```python
from build123d import *

# Parameters (mm, degrees)
SALIENTE_EXTRUIR1_DEPTH = 0.8
CROQUIS5_R              = 5.15
CORTAR_EXTRUIR1_DEPTH   = 0.8
CROQUIS4_R              = 2.1
CORTAR_EXTRUIR2_DEPTH   = 0.8


with BuildPart() as part:
    # Croquis1 → Saliente-Extruir1 (new body)
    with BuildSketch(Plane.XY):
        with BuildLine():
            Line((-55.5, 86), (-55.5, 78))
            ThreePointArc((-55.5, 78), (-55.792893219, 77.292893219), (-56.5, 77))
            Line((-56.5, 77), (-58.5, 77))
            ThreePointArc((-58.5, 77), (-59.207106781, 76.707106781), (-59.5, 76))
            Line((-59.5, 76), (-59.5, -36))
            ThreePointArc((-59.5, -36), (-58.621320344, -38.121320344), (-56.5, -39))
            Line((-56.5, -39), (50.5, -39))
            ThreePointArc((50.5, -39), (52.621320344, -38.121320344), (53.5, -36))
            Line((53.5, -36), (53.5, 124))
            ThreePointArc((53.5, 124), (52.621320344, 126.121320344), (50.5, 127))
            Line((50.5, 127), (-56.5, 127))
            ThreePointArc((-56.5, 127), (-58.621320344, 126.121320344), (-59.5, 124))
            Line((-59.5, 124), (-59.5, 88))
            ThreePointArc((-59.5, 88), (-59.207106781, 87.292893219), (-58.5, 87))
            Line((-58.5, 87), (-56.5, 87))
            ThreePointArc((-56.5, 87), (-55.792893219, 86.707106781), (-55.5, 86))
        make_face()
    extrude(amount=SALIENTE_EXTRUIR1_DEPTH)

    # Croquis5 → Cortar-Extruir1 (cut)
    with BuildSketch(Plane.XY.offset(0.8)):
        Circle(CROQUIS5_R)
        with BuildLine():
            Line((-17.937391115, -1.5), (-12.787322824, -1.5))
            ThreePointArc((-12.787322824, -1.5), (-9.103999808, -9.103999808), (-1.5, -12.787322824))
            Line((-1.5, -12.787322824), (-1.5, -17.937391115))
            ThreePointArc((-1.5, -17.937391115), (-12.727922061, -12.727922061), (-17.937391115, -1.5))
        make_face()
        with BuildLine():
            Line((-17.937391115, 1.5), (-12.787322824, 1.5))
            ThreePointArc((-12.787322824, 1.5), (-9.103999808, 9.103999808), (-1.5, 12.787322824))
            Line((-1.5, 12.787322824), (-1.5, 17.937391115))
            ThreePointArc((-1.5, 17.937391115), (-12.727922061, 12.727922061), (-17.937391115, 1.5))
        make_face()
        with BuildLine():
            Line((1.5, -17.937391115), (1.5, -12.787322824))
            ThreePointArc((1.5, -12.787322824), (9.103999808, -9.103999808), (12.787322824, -1.5))
            Line((12.787322824, -1.5), (17.937391115, -1.5))
            ThreePointArc((17.937391115, -1.5), (12.727922061, -12.727922061), (1.5, -17.937391115))
        make_face()
        with BuildLine():
            Line((-10.139649895, 1.5), (-7.603453163, 1.5))
            ThreePointArc((-7.603453163, 1.5), (-5.480077554, 5.480077554), (-1.5, 7.603453163))
            Line((-1.5, 7.603453163), (-1.5, 10.139649895))
            ThreePointArc((-1.5, 10.139649895), (-7.247844507, 7.247844507), (-10.139649895, 1.5))
        make_face()
        with BuildLine():
            Line((-10.139649895, -1.5), (-7.603453163, -1.5))
            ThreePointArc((-7.603453163, -1.5), (-5.480077554, -5.480077554), (-1.5, -7.603453163))
            Line((-1.5, -7.603453163), (-1.5, -10.139649895))
            ThreePointArc((-1.5, -10.139649895), (-7.247844507, -7.247844507), (-10.139649895, -1.5))
        make_face()
        with BuildLine():
            Line((7.603453163, -1.5), (10.139649895, -1.5))
            ThreePointArc((10.139649895, -1.5), (7.247844507, -7.247844507), (1.5, -10.139649895))
            Line((1.5, -10.139649895), (1.5, -7.603453163))
            ThreePointArc((1.5, -7.603453163), (5.480077554, -5.480077554), (7.603453163, -1.5))
        make_face()
        with BuildLine():
            Line((7.603453163, 1.5), (10.139649895, 1.5))
            ThreePointArc((10.139649895, 1.5), (7.247844507, 7.247844507), (1.5, 10.139649895))
            Line((1.5, 10.139649895), (1.5, 7.603453163))
            ThreePointArc((1.5, 7.603453163), (5.480077554, 5.480077554), (7.603453163, 1.5))
        make_face()
        with BuildLine():
            Line((12.787322824, 1.5), (17.937391115, 1.5))
            ThreePointArc((17.937391115, 1.5), (12.727922061, 12.727922061), (1.5, 17.937391115))
            Line((1.5, 17.937391115), (1.5, 12.787322824))
            ThreePointArc((1.5, 12.787322824), (9.103999808, 9.103999808), (12.787322824, 1.5))
        make_face()
    extrude(amount=-CORTAR_EXTRUIR1_DEPTH, mode=Mode.SUBTRACT)

    # Croquis4 → Cortar-Extruir2 (cut)
    with BuildSketch(Plane.XY.offset(0.8)):
        with Locations((-54.5, -31.5)):
            Circle(CROQUIS4_R)
        with Locations((48.5, -31.5)):
            Circle(CROQUIS4_R)
        with BuildLine():
            Line((-6.348885271, 98.8), (1.5, 98.8))
            ThreePointArc((1.5, 98.8), (3.3, 97), (1.5, 95.2))
            Line((1.5, 95.2), (-6.348885271, 95.2))
            ThreePointArc((-6.348885271, 95.2), (-8.148885271, 97), (-6.348885271, 98.8))
        make_face()
    extrude(amount=-CORTAR_EXTRUIR2_DEPTH, mode=Mode.SUBTRACT)


solid = part.part
```
The listing builds one solid part. Answer for the finished solid, in the listing's coordinates (mm). A direction names the side the tool comes from. Coordinates: 2 decimals unless noted, no trailing zeros. Write each loop counter-clockwise with the first axis right and the second up, starting at its lowest first coordinate (ties: lowest second). Pieces come first, ordered by that corner, then holes. Notation, with made-up numbers: (-9.5, -38) - (45.5, -38) arc R35 cw to (45.5, 1) - close; hole circle Ø5 at (14, -23.75). An arc over 180 degrees is marked (long way). Return JSON: item names as keys, results as strings. Group by question number.
1. A cutting plane is placed at A-A, the plane y = 97. Determine the outline of the cut face in (x, z), plus the area to 3 significant figures.
2. A cutting plane is placed at B-B, the plane x = 48.5. Determine the outline of the cut face in (y, z).
3. A cutting plane is placed at C-C, the plane y = -31.5. Determine the outline of the cut face in (x, z).
4. A cutting plane is placed at D-D, the plane z = 0.6. Give the number of separate pieces and of enclosed holes in the cut face, plus the area to 3 significant figures.
5. Which of the six approach directions +Z, -Z, +X, -X, +Y, -Y give full straight-line access (tool end or side, diameter ignored) to faces 4 (the cylindrical face through (-5.53, -5.43, 0.41)), 5 (the flat face through (-4, 45, 0))?
6. Straight lines are drawn through the part: L1, parallel to Y at x = 0, z = 0.55; L2, parallel to Y at x = 48.5, z = 0.45; L3, parallel to Y at x = 16.5, z = 0.2. For each, find the intervals that lie inside material, in ascending order.
7. Determine the mould class of faces 1 (the cylindrical face through (-7.183, 7.312, 0.406)), 2 (the cylindrical face through (9.02, -9.19, 0.41)), 3 (the flat face through (-4, 45, 0.8)) for opening direction Y: released by +Y, released by -Y, zero draft, split by the parting line, or undercut.
Ans:
{
 "1": {"outline": "(-59.5, 0) - (-8.15, 0) - (-8.15, 0.8) - (-59.5, 0.8) - close; (3.3, 0) - (53.5, 0) - (53.5, 0.8) - (3.3, 0.8) - close", "area": "81.2 mm²"},
 "2": {"outline": "(-39, 0) - (-33.6, 0) - (-33.6, 0.8) - (-39, 0.8) - close; (-29.4, 0) - (127, 0) - (127, 0.8) - (-29.4, 0.8) - close"},
 "3": {"outline": "(-59.5, 0) - (-56.6, 0) - (-56.6, 0.8) - (-59.5, 0.8) - close; (-52.4, 0) - (46.4, 0) - (46.4, 0.8) - (-52.4, 0.8) - close; (50.6, 0) - (53.5, 0) - (53.5, 0.8) - (50.6, 0.8) - close"},
 "4": {"separate pieces": "1", "enclosed holes": "12", "area": "18,000 mm²"},
 "5": {"face 4": "+Z, -Z", "face 5": "-Z, +X, -X, +Y, -Y"},
 "6": {"L1": "-39 to -5.15, 5.15 to 95.2, 98.8 to 127", "L2": "-39 to -33.6, -29.4 to 127", "L3": "-39 to -7.19, -1.5 to 1.5, 7.19 to 127"},
 "7": {"face 1": "undercut", "face 2": "undercut", "face 3": "zero draft"}
}
